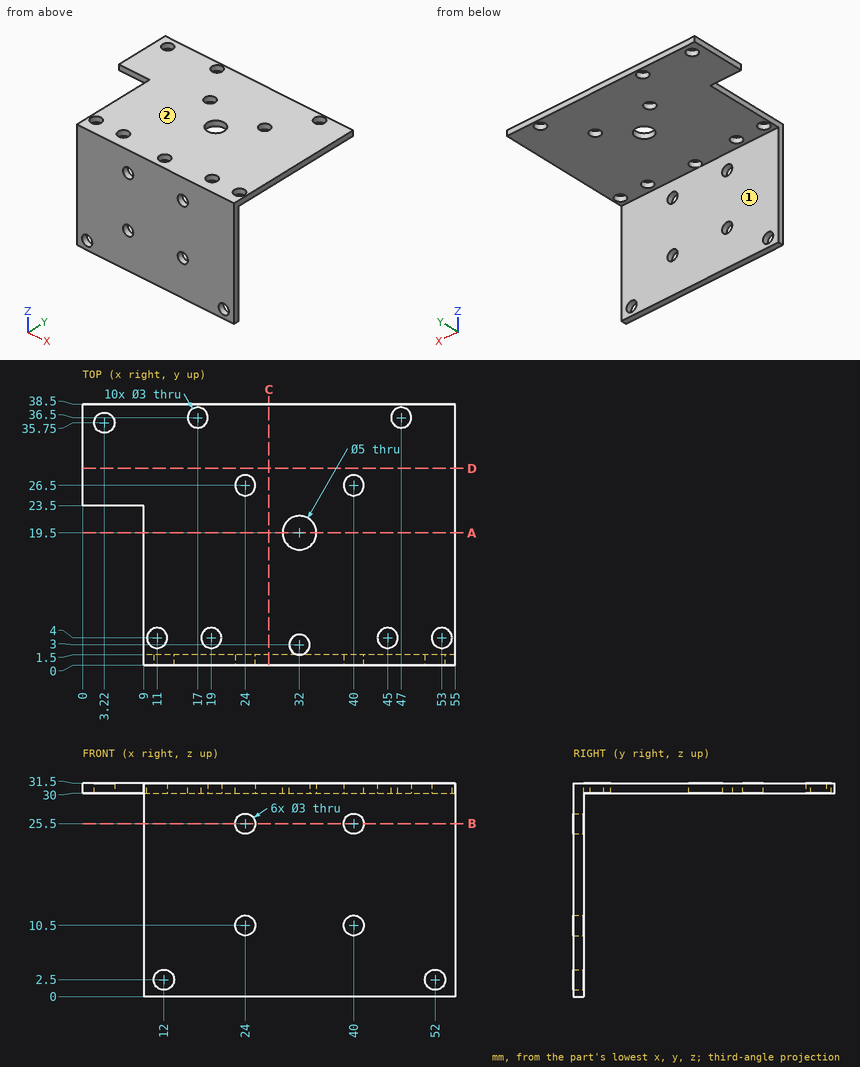
Could you check a few things on this drawing? It's one solid part, dimensions in mm from its lowest x, y, z. A direction names the side the tool comes from. Round coordinates to 2 decimals unless told otherwise and drop trailing zeros. Order: outer loops, then holes, each group sorted by start corner. A loop starts at its lowest first (then second) coordinate and runs counter-clockwise, first axis right, second up. Notation, with made-up numbers: M 66.25,-39 L 83.25,-39 A22 cw 83.25,-28 Z; hole C 36.5,78.5 d9. An arc over 180 degrees is marked long. One line per question, with ' | ' between items. Start each with the question number.
(1) Suppose I cut it at A-A on y = 19.5. List the corners of the cut face in (x, z) for me.
(2) Please list where these lines run through material, in increasing order: line 1 along Z through (x, y) = (40, 1.15); line 2 along Z through (x, y) = (52, 0.9); line 3 along Y through (x, z) = (47, 31).
(3) Suppose I cut it at C-C on x = 27.5. List the corners of the cut face in (y, z) for me, then the cut area to 3 significant figures.
(4) Suppose I cut it at D-D on y = 29. List the corners of the cut face in (x, z) for me, then the cut area to 3 significant figures.
(5) Suppose I cut it at B-B on z = 25.5. List the corners of the cut face in (x, y) for me.
(6) For P1, Ø4, axis at x = 17, y = 36.5, coming from the -Z side; P2, Ø3.5, axis at x = 12, z = 2.5, coming from the +Y side; P3, Ø0.8, axis at x = 3, z = 31, coming from the -Y side, each with a flat end and sliding along its axis, tell me the tip position at first contact or that it passes through.
(7) For the marked faces 1 and 2, which set-ups out of +Z, -Z, +X, -X, +Y, -Y let a thin tool reach every point of the face, with its end or its side?
Geometry results:
1) outline: M 9,30 L 29.5,30 L 29.5,31.5 L 9,31.5 Z; M 34.5,30 L 55,30 L 55,31.5 L 34.5,31.5 Z
2) line 1: 0 to 9, 12 to 24, 27 to 31.5 | line 2: 0 to 1, 4 to 31.5 | line 3: 0 to 35, 38 to 38.5
3) outline: M 0,0 L 1.5,0 L 1.5,30 L 38.5,30 L 38.5,31.5 L 0,31.5 Z | area: 103 mm²
4) outline: M 0,30 L 55,30 L 55,31.5 L 0,31.5 Z | area: 82.5 mm²
5) outline: M 9,0 L 22.5,0 L 22.5,1.5 L 9,1.5 Z; M 25.5,0 L 38.5,0 L 38.5,1.5 L 25.5,1.5 Z; M 41.5,0 L 55,0 L 55,1.5 L 41.5,1.5 Z
6) P1: z = 30 | P2: y = 1.5 | P3: y = 23.5
7) face 1: -Z, +X, -X, +Y | face 2: +Z, +X, -X, +Y, -Y
